The model under review builds one solid part; all positions refer to its coordinate system, in mm. Face numbers are marked on the shaded views. A direction names the side the tool comes from. Give positions to 0.01 mm unless a question says otherwise; leave off trailing zeros. Loops run counter-clockwise (first coordinate to the right, second up) from the corner with the lowest first, then second, coordinate; pieces in that order, holes last. Notation, with made-up numbers: (56, -10.75) -> (92, -10.75) arc R10 cw to (92, 2.25) -> close; hole circle Ø6 at (-14.75, -26). An arc over 180 degrees is marked (long way). Write each question's results on one line, items separated by ' | '. Start each with the question number.
Q1. Machinability: for the marked faces 1, 2 and 3, which of the approach directions +Z, -Z, +X, -X, +Y, -Y give a long, thin tool a straight path to every point of the face, cutting with its end or side? Answer none if there is none.
Q2. We need section C-C (z = 55.5). Write out the cut boundary in (x, y), plus the area to 3 significant figures.
Q3. Wall thickness on L1, parallel to X at y = -23, z = 54.5; L2, parallel to Y at x = -18.5, z = 52.75; L3, parallel to X at y = -27, z = 54: over which ranges is each line inside the solid? List them lowest first. Write a range as [from, to].
Q4. Mouldability with a two-part tool opening along Y and no side actions: class the marked faces 4, 5, 6 and 7 as released by +Y, released by -Y, zero draft, split by the parting line, or undercut.
Q5. Insertion check: pin 1 Ø4 at (x, z) = (-31.72, 55.12) entering from +Y; pin 2 Ø1.5 at (y, z) = (-45, 56) entering from -X; pin 3 Ø2 at (y, z) = (-42, 56.5) entering from +X. Each pin has a flat end and moves straight along its axis. Give the tip position at first contact, or say it passes through.
Q6. We need section A-A (x = -20.75). Write out the cut boundary in (y, z), plus the area to 3 significant figures.
Q7. We need section B-B (x = -17.25). Write out the cut boundary in (y, z).
Q8. We need section D-D (y = -23.5). Write out the cut boundary in (x, z), plus the area to 3 significant figures.
from build123d import *

# Parameters (mm, degrees)
SKETCH2_W                      = 6.7
SKETCH2_H                      = 3
BOSS_EXTRUDE1_DEPTH            = 12.100000416
BOSS_EXTRUDE1_2_DEPTH          = 12.100000416
BOSS_EXTRUDE2_START            = -12.1
SKETCH2_3_W                    = 6.7
SKETCH2_3_H                    = 3
SKETCH2_3_H_2                  = 29.35460187
BOSS_EXTRUDE2_DEPTH            = 4
CUT_EXTRUDE1_REACH             = 78.977
SKETCH3_R                      = 1.6
CUT_EXTRUDE1_DIRECTION_2_DEPTH = 77.976712266
BOSS_EXTRUDE4_START            = -16.100002
SKETCH2_4_W                    = 6.7
SKETCH2_4_H                    = 3
BOSS_EXTRUDE4_DEPTH            = 7
CUT_EXTRUDE2_REACH             = 78.977
SKETCH6_R                      = 1.6
CUT_EXTRUDE2_DIRECTION_2_DEPTH = 77.976712266


with BuildPart() as part:
    # Sketch2 → Boss-Extrude1 (new body)
    with BuildSketch(Plane.ZY.offset(37.766138352)):
        with Locations((55.120130346, -55.592329425)):
            Rectangle(SKETCH2_W, SKETCH2_H)
    extrude(amount=-BOSS_EXTRUDE1_DEPTH)



with BuildPart() as body_2:
    # Sketch2 → Boss-Extrude1 2 (new body)
    with BuildSketch(Plane.ZY.offset(37.766138352)):
        Polygon((51.770130346, -21.737727555), (51.770130346, -24.737727555), (58.470130346, -24.737727555), (58.470130346, -21.223242389), align=None)
    extrude(amount=-BOSS_EXTRUDE1_2_DEPTH)


with BuildPart() as part_1:
    add(part.part)

    add(body_2.part)  # Boss-Extrude2 merges body 2
    # Sketch2<3> → Boss-Extrude2 (add)
    with BuildSketch(Plane.ZY.offset(37.766138352).offset(BOSS_EXTRUDE2_START)):
        with Locations((55.120130346, -55.592329425)):
            Rectangle(SKETCH2_3_W, SKETCH2_3_H)
        with Locations((55.120130346, -39.41502849)):
            Rectangle(SKETCH2_3_W, SKETCH2_3_H_2)
        Polygon((51.770130346, -21.737727555), (51.770130346, -24.737727555), (58.470130346, -24.737727555), (58.470130346, -21.223242389), align=None)
    extrude(amount=-BOSS_EXTRUDE2_DEPTH)

    # Sketch3 → Cut-Extrude1 (cut, up to next)
    with BuildSketch(Plane(origin=(0, -54.092329425, 0), x_dir=(1, 0, 0), z_dir=(0, 1, 0)), mode=Mode.PRIVATE) as cut_extrude1_sk1:
        with Locations(Location((-31.716139041, -55.120130346, 0), (0, 0, 180))):
            Circle(SKETCH3_R)
    cut_extrude1_tool1 = extrude(cut_extrude1_sk1.sketch, amount=-CUT_EXTRUDE1_REACH, mode=Mode.PRIVATE) & part_1.part
    add(cut_extrude1_tool1.solids().sort_by_distance((-31.716139, -54.092329, 55.12013))[0], mode=Mode.SUBTRACT)

    # Sketch3 → Cut-Extrude1 direction 2 (cut)
    with BuildSketch(Plane(origin=(0, -54.092329425, 0), x_dir=(1, 0, 0), z_dir=(0, 1, 0))):
        with Locations(Location((-31.716139041, -55.120130346, 0), (0, 0, 180))):
            Circle(SKETCH3_R)
    extrude(amount=CUT_EXTRUDE1_DIRECTION_2_DEPTH, mode=Mode.SUBTRACT)


with BuildPart() as boss_extrude4_tool:
    # Sketch2<4> → Boss-Extrude4 (new body)
    with BuildSketch(Plane.ZY.offset(37.766138352).offset(BOSS_EXTRUDE4_START)):
        with Locations((55.120130346, -55.592329425)):
            Rectangle(SKETCH2_4_W, SKETCH2_4_H)
        Polygon((51.770130346, -21.737727555), (51.770130346, -24.737727555), (58.470130346, -24.737727555), (58.470130346, -21.223242389), align=None)
    extrude(amount=-BOSS_EXTRUDE4_DEPTH)


with BuildPart() as part_2:
    add(part_1.part)


with BuildPart() as part_3:
    # Boss-Extrude4: joined with boss_extrude4_tool
    add(part_2.part.fuse(boss_extrude4_tool.part, tol=0.00001))

    # Sketch6 → Cut-Extrude2 (cut, up to next)
    with BuildSketch(Plane(origin=(0, -54.092329425, 0), x_dir=(1, 0, 0), z_dir=(0, 1, 0)), mode=Mode.PRIVATE) as cut_extrude2_sk1:
        with Locations(Location((-18.166139731, -55.120130346, 0), (0, 0, 90))):
            Circle(SKETCH6_R)
    cut_extrude2_tool1 = extrude(cut_extrude2_sk1.sketch, amount=-CUT_EXTRUDE2_REACH, mode=Mode.PRIVATE) & part_3.part
    add(cut_extrude2_tool1.solids().sort_by_distance((-18.16614, -54.092329, 55.12013))[0], mode=Mode.SUBTRACT)

    # Sketch6 → Cut-Extrude2 direction 2 (cut)
    with BuildSketch(Plane(origin=(0, -54.092329425, 0), x_dir=(1, 0, 0), z_dir=(0, 1, 0))):
        with Locations(Location((-18.166139731, -55.120130346, 0), (0, 0, 90))):
            Circle(SKETCH6_R)
    extrude(amount=CUT_EXTRUDE2_DIRECTION_2_DEPTH, mode=Mode.SUBTRACT)


solid = part_3.part
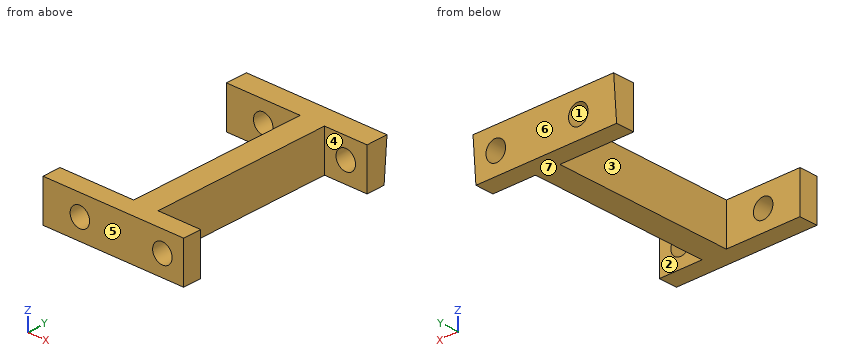
Output:
1) face 1: +Y, -Y | face 2: +Z, -Z, +X | face 3: +Z, -Z, -X
2) outline: (-37.77, -57.09) -> (-33.27, -57.09) -> (-33.27, -54.09) -> (-37.77, -54.09) -> close; (-37.77, -24.74) -> (-33.27, -24.74) -> (-33.27, -21.45) -> (-37.77, -21.45) -> close; (-30.16, -57.09) -> (-19.72, -57.09) -> (-19.72, -54.09) -> (-21.67, -54.09) -> (-21.67, -24.74) -> (-19.72, -24.74) -> (-19.72, -21.45) -> (-30.16, -21.45) -> (-30.16, -24.74) -> (-25.67, -24.74) -> (-25.67, -54.09) -> (-30.16, -54.09) -> close; (-16.61, -57.09) -> (-14.67, -57.09) -> (-14.67, -54.09) -> (-16.61, -54.09) -> close; (-16.61, -24.74) -> (-14.67, -24.74) -> (-14.67, -21.45) -> (-16.61, -21.45) -> close | area: 224 mm2
3) L1: [-37.77, -33.19], [-30.24, -19.64], [-16.69, -14.67] | L2: [-57.09, -54.09], [-24.74, -21.66] | L3: [-25.67, -21.67]
4) face 4: undercut | face 5: released by -Y | face 6: released by +Y | face 7: zero draft
5) pin 1: y = -21.33 | pin 2: x = -25.67 | pin 3: x = -21.67
6) outline: (-57.09, 51.77) -> (-54.09, 51.77) -> (-54.09, 58.47) -> (-57.09, 58.47) -> close; (-24.74, 51.77) -> (-21.74, 51.77) -> (-21.22, 58.47) -> (-24.74, 58.47) -> close | area: 41.9 mm2
7) outline: (-57.09, 51.77) -> (-54.09, 51.77) -> (-54.09, 53.81) -> (-57.09, 53.81) -> close; (-57.09, 56.43) -> (-54.09, 56.43) -> (-54.09, 58.47) -> (-57.09, 58.47) -> close; (-24.74, 51.77) -> (-21.74, 51.77) -> (-21.58, 53.81) -> (-24.74, 53.81) -> close; (-24.74, 56.43) -> (-21.38, 56.43) -> (-21.22, 58.47) -> (-24.74, 58.47) -> close
8) outline: (-37.77, 51.77) -> (-14.67, 51.77) -> (-14.67, 58.47) -> (-37.77, 58.47) -> close; hole circle Ø3.2 at (-31.72, 55.12); hole circle Ø3.2 at (-18.17, 55.12) | area: 139 mm2
